For this review, take the finished solid that the model builds, in its own axes (mm). Give positions to 0.01 mm unless a question says otherwise; leave off trailing zeros. Write each loop counter-clockwise with the first axis right and the second up, starting at its lowest first coordinate (ties: lowest second). Pieces come first, ordered by that corner, then holes. Notation, with made-up numbers: (61, 46.5) -> (100, 46.5) arc R12 cw to (100, 69.5) -> close; hole circle Ø9 at (8.5, 66.5). An arc over 180 degrees is marked (long way). Write item = value, one per line.
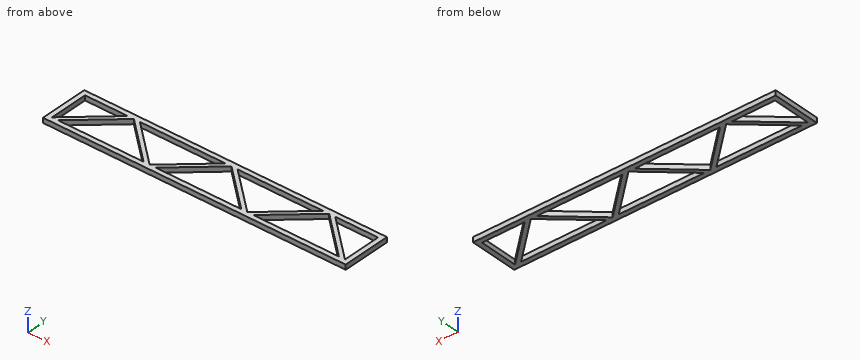
```python
from build123d import *

# Parameters (mm, degrees)
SKETCH_1_W      = 250
SKETCH_1_H      = 40
SKETCH_1_W_2    = 242
SKETCH_1_H_2    = 32
EXTRUDE_1_DEPTH = 4


with BuildPart() as part:
    # 草图1 → 凸台-拉伸1 (new body)
    # profile 1 of 7: a face of its own
    with BuildSketch(Plane.XY):
        Rectangle(SKETCH_1_W, SKETCH_1_H)
        Rectangle(SKETCH_1_W_2, SKETCH_1_H_2, mode=Mode.SUBTRACT)
    # profile 2 of 7: a face of its own
    with BuildSketch(Plane.XY):
        Polygon((-80.666666667, 16), (-85.666666667, 16), (-121, -16), (-116, -16), align=None)
    # profile 3 of 7: a face of its own
    with BuildSketch(Plane.XY):
        Polygon((-75.666666667, 16), (-80.666666667, 16), (-45.333333333, -16), (-40.333333333, -16), align=None)
    # profile 4 of 7: a face of its own
    with BuildSketch(Plane.XY):
        Polygon((0, 16), (-5, 16), (-40.333333333, -16), (-35.333333333, -16), align=None)
    # profile 5 of 7: a face of its own
    with BuildSketch(Plane.XY):
        Polygon((5, 16), (0, 16), (35.333333333, -16), (40.333333333, -16), align=None)
    # profile 6 of 7: a face of its own
    with BuildSketch(Plane.XY):
        Polygon((80.666666667, 16), (75.666666667, 16), (40.333333333, -16), (45.333333333, -16), align=None)
    # profile 7 of 7: a face of its own
    with BuildSketch(Plane.XY):
        Polygon((85.666666667, 16), (80.666666667, 16), (116, -16), (121, -16), align=None)
    extrude(amount=EXTRUDE_1_DEPTH)


solid = part.part
```
(1) Take a section at A-A (z = 2.4). Write out the cut boundary in (x, y).
Answers below:
outline = (-125, -20) -> (125, -20) -> (125, 20) -> (-125, 20) -> close; hole (-121, -16) -> (-85.67, 16) -> (-121, 16) -> close; hole (-116, -16) -> (-45.33, -16) -> (-80.67, 16) -> close; hole (-75.67, 16) -> (-40.33, -16) -> (-5, 16) -> close; hole (-35.33, -16) -> (35.33, -16) -> (0, 16) -> close; hole (5, 16) -> (40.33, -16) -> (75.67, 16) -> close; hole (45.33, -16) -> (116, -16) -> (80.67, 16) -> close; hole (85.67, 16) -> (121, -16) -> (121, 16) -> close
(2) Take a section at C-C (x = 10). Write out the cut boundary in (y, z), plus the area to 3 significant figures.
Answers below:
outline = (-20, 0) -> (-16, 0) -> (-16, 4) -> (-20, 4) -> close; (6.94, 0) -> (11.47, 0) -> (11.47, 4) -> (6.94, 4) -> close; (16, 0) -> (20, 0) -> (20, 4) -> (16, 4) -> close
area = 50.1 mm^2
(3) To check wall thickness, follow probe 1 along Y at (x, z) = (100, 1.05); probe 2 along Y at (x, z) = (87, 1.65). State the ranges of each line that lie inside material, in increasing order.
Answers below:
probe_1 = -20 to -16, -1.51 to 3.02, 16 to 20
probe_2 = -20 to -16, 10.26 to 14.79, 16 to 20
(4) Take a section at B-B (y = -3.5). Count the separate pieces of the cut face and the enclosed holes in it, plus the area to 3 significant figures.
Answers below:
separate_pieces = 8
enclosed_holes = 0
area = 152 mm^2
